For this review, take the finished solid that the model builds, in its own axes (mm). Face numbers are marked on the shaded views. A direction names the side the tool comes from. Give positions to 0.01 mm unless a question says otherwise; leave off trailing zeros. Order: outer loops, then holes, each group sorted by start corner. A loop starts at its lowest first (then second) coordinate and runs counter-clockwise, first axis right, second up. Notation, with made-up numbers: (-28, 88) - (12, 88) arc R32 cw to (12, 116) - close; hole circle Ø11 at (42, 77). An arc over 180 degrees is marked (long way). Use a Markdown table: item, result. Add a question column.
1) Wall thickness on L1, parallel to Y at x = -82.55, z = 2.75; L2, parallel to X at y = -82, z = 1; L3, parallel to Y at x = 7, z = 638: over which ranges is each line inside the solid? List them lowest first.
2) Machinability: for the marked faces 1, 2 and 3, which of the approach directions +Z, -Z, +X, -X, +Y, -Y give a long, thin tool a straight path to every point of the face, cutting with its end or side? Answer none if there is none.
3) Clearance check with flat-ended pins moving along their axes: P1, Ø21, axis at y = -8.5, z = 423, coming from the +X side; P2, Ø1.5, axis at x = 32.5, y = 52, coming from the +Z side; P3, Ø5, axis at x = 37.5, z = 96, coming from the +Y side. State where each tip first meets the part, or that it passes through.
4) We need section D-D on y = 67.5. Write out the cut boundary in (x, z).
5) We need section B-B on x = -3. Write out the cut boundary in (y, z), then the cut area to 3 significant figures.
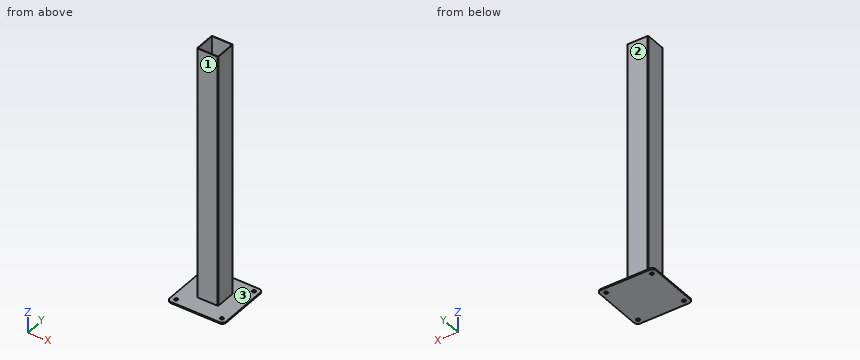
```python
from build123d import *

# Parameters (mm, degrees)
F0_W     = 203.2
F0_H     = 203.2
F0_R     = 6.35
F1_DEPTH = 4.7625
F2_R     = 12.7
F4_DEPTH = 914.4


with BuildPart() as f1:
    # F0 (on Top) → F1 (new body)
    with BuildSketch(Plane.XY):
        Rectangle(F0_W, F0_H)
        with Locations((-82.55, -82.55)):
            Circle(F0_R, mode=Mode.SUBTRACT)
        with Locations((82.55, -82.55)):
            Circle(F0_R, mode=Mode.SUBTRACT)
        with Locations((-82.55, 82.55)):
            Circle(F0_R, mode=Mode.SUBTRACT)
        with Locations((82.55, 82.55)):
            Circle(F0_R, mode=Mode.SUBTRACT)
    extrude(amount=F1_DEPTH)

    # F2
    f2_edges = [f1.edges().sort_by_distance(p)[0] for p in [
        (-101.6, -101.6, 2.38125),
        (101.6, -101.6, 2.38125),
        (101.6, 101.6, 2.38125),
        (-101.6, 101.6, 2.38125),
    ]]
    fillet(f2_edges, radius=F2_R)

    # F3 (on face) → F4 (join)
    with BuildSketch(Plane.XY.offset(4.7625)):
        with BuildLine():
            Line((34.925, 38.1), (-34.925, 38.1))
            ThreePointArc((-34.925, 38.1), (-37.170064, 37.170064), (-38.1, 34.925))
            Line((-38.1, 34.925), (-38.1, -34.925))
            ThreePointArc((-38.1, -34.925), (-37.170064, -37.170064), (-34.925, -38.1))
            Line((-34.925, -38.1), (34.925, -38.1))
            ThreePointArc((34.925, -38.1), (37.170064, -37.170064), (38.1, -34.925))
            Line((38.1, -34.925), (38.1, 34.925))
            ThreePointArc((38.1, 34.925), (37.170064, 37.170064), (34.925, 38.1))
        make_face()
        with BuildLine():
            Line((-36.5125, -34.925), (-36.5125, 34.925))
            ThreePointArc((-36.5125, 34.925), (-36.047532, 36.047532), (-34.925, 36.5125))
            Line((-34.925, 36.5125), (34.925, 36.5125))
            ThreePointArc((34.925, 36.5125), (36.047532, 36.047532), (36.5125, 34.925))
            Line((36.5125, 34.925), (36.5125, -34.925))
            ThreePointArc((36.5125, -34.925), (36.047532, -36.047532), (34.925, -36.5125))
            Line((34.925, -36.5125), (-34.925, -36.5125))
            ThreePointArc((-34.925, -36.5125), (-36.047532, -36.047532), (-36.5125, -34.925))
        make_face(mode=Mode.SUBTRACT)
    extrude(amount=F4_DEPTH)


solid = f1.part
```
Checked values:
| question | item | result |
|---|---|---|
| 1 | L1 | -101.6 to -88.9, -76.2 to 76.2, 88.9 to 101.6 |
| 1 | L2 | -101.6 to -88.88, -76.22 to 76.22, 88.88 to 101.6 |
| 1 | L3 | -38.1 to -36.51, 36.51 to 38.1 |
| 2 | face 1 | +Z, +X, -X, -Y |
| 2 | face 2 | +Z, +X, -X, +Y |
| 2 | face 3 | +Z |
| 3 | P1 | x = 38.1 |
| 3 | P2 | z = 4.76 |
| 3 | P3 | y = 38.1 |
| 4 | outline | (-101.6, 0) - (101.6, 0) - (101.6, 4.76) - (-101.6, 4.76) - close |
| 5 | outline | (-101.6, 0) - (101.6, 0) - (101.6, 4.76) - (38.1, 4.76) - (38.1, 919.16) - (36.51, 919.16) - (36.51, 4.76) - (-36.51, 4.76) - (-36.51, 919.16) - (-38.1, 919.16) - (-38.1, 4.76) - (-101.6, 4.76) - close |
| 5 | area | 3,870 mm² |
